Part print with two shaded views. Sizes in mm from the minimum x, y, z corner. Round coordinates to 2 decimals unless told otherwise and drop trailing zeros. Loops run counter-clockwise (first coordinate to the right, second up) from the corner with the lowest first, then second, coordinate; pieces in that order, holes last. Notation, with made-up numbers: (6, 84.25) -> (22, 84.25) arc R28 ccw to (22, 108.25) -> close; hole circle Ø7 at (30.5, 53). An arc over 180 degrees is marked (long way). Use a Markdown table: item, result. Add a question column.
Item 1: Cut at B-B, the plane x = 5.25. List the corners of the cut face in (y, z), plus the area to 3 significant figures.
Item 2: Flat gauge pin, fed straight in: pin 1 (7.5 mm diameter, centred on x = 9.525, y = 9.525, fed in from +Z). Where does the tip first touch, or does it go through?
Item 3: Probe line 1 (X direction, y = 12.5, z = 13); line 2 (X direction, y = 10, z = 18); line 3 (Y direction, x = 5.5, z = 18.25). List the from-to ranges inside material, lowest first. Write a range as [from, to].
Item 4: Two-plate mould, pull along X, no slides. Class the marked faces 1, 2 and 3: pulls with the +X half, pulls with the -X half, needs draft (parallel to the pull), parting line crosses it, or undercut.
Item 5: Cut at A-A, the plane y = 13. List the corners of the cut face in (x, z).
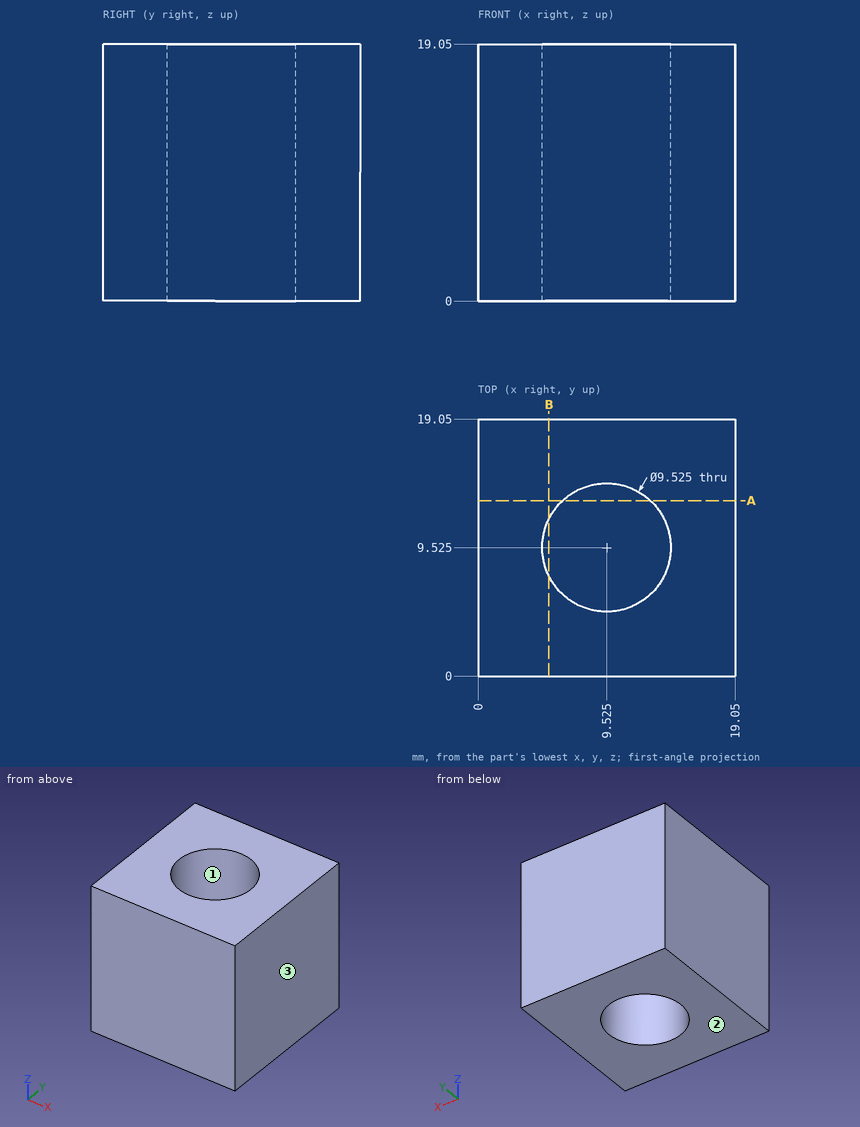
A:
| question | item | result |
|---|---|---|
| 1 | outline | (0, 0) -> (7.43, 0) -> (7.43, 19.05) -> (0, 19.05) -> close; (11.62, 0) -> (19.05, 0) -> (19.05, 19.05) -> (11.62, 19.05) -> close |
| 1 | area | 283 mm^2 |
| 2 | pin 1 | passes through |
| 3 | line 1 | x = [0, 5.81], [13.24, 19.05] |
| 3 | line 2 | x = [0, 4.79], [14.26, 19.05] |
| 3 | line 3 | y = [0, 6.98], [12.07, 19.05] |
| 4 | face 1 | undercut |
| 4 | face 2 | needs draft |
| 4 | face 3 | pulls with the +X half |
| 5 | outline | (0, 0) -> (6.27, 0) -> (6.27, 19.05) -> (0, 19.05) -> close; (12.78, 0) -> (19.05, 0) -> (19.05, 19.05) -> (12.78, 19.05) -> close |
